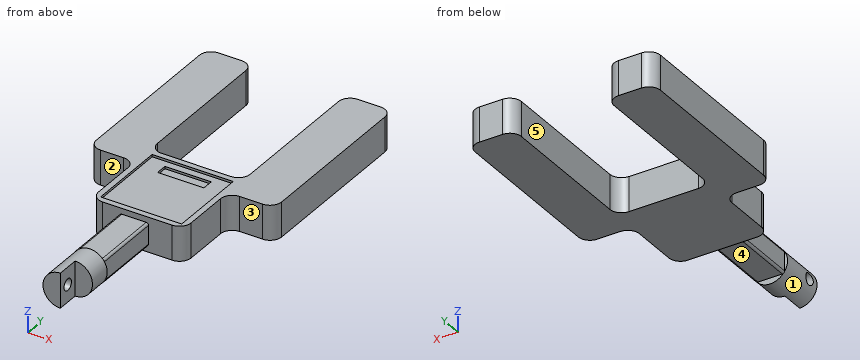
from build123d import *

# Parameters (mm, degrees)
SKETCH1_W           = 101.6
SKETCH1_H           = 101.6
BOSS_EXTRUDE1_DEPTH = 38.1
SKETCH2_W           = 50.8
SKETCH2_H           = 12.7
CUT_EXTRUDE1_DEPTH  = 5.08
SKETCH3_W           = 88.9
SKETCH3_H           = 88.9
CUT_EXTRUDE2_DEPTH  = 2.54
SKETCH4_W           = 31.75
SKETCH4_H           = 25.4
BOSS_EXTRUDE2_DEPTH = 76.2
SKETCH6_R           = 19.05
BOSS_EXTRUDE3_DEPTH = 50.8
SKETCH7_W           = 24.863041021
SKETCH7_H           = 49.917211664
CUT_EXTRUDE3_DEPTH  = 25.4
SKETCH8_W           = 50.8
SKETCH8_H           = 203.2
BOSS_EXTRUDE4_DEPTH = 38.1
FILLET1_R           = 12.7
SKETCH9_R           = 6.35
CUT_EXTRUDE4_DEPTH  = 301.990708903
FILLET2_R           = 2.54


with BuildPart() as part:
    # Sketch1 → Boss-Extrude1 (new body)
    with BuildSketch(Plane.XY):
        with Locations((50.8, 50.8)):
            Rectangle(SKETCH1_W, SKETCH1_H)
    extrude(amount=BOSS_EXTRUDE1_DEPTH)

    # Sketch2 → Cut-Extrude1 (cut)
    with BuildSketch(Plane.XY.offset(38.1)):
        with Locations((50.8, 80.942159742)):
            Rectangle(SKETCH2_W, SKETCH2_H)
    extrude(amount=-CUT_EXTRUDE1_DEPTH, mode=Mode.SUBTRACT)

    # Sketch3 → Cut-Extrude2 (cut)
    with BuildSketch(Plane.XY.offset(38.1)):
        with Locations((50.8, 50.8)):
            Rectangle(SKETCH3_W, SKETCH3_H)
    extrude(amount=-CUT_EXTRUDE2_DEPTH, mode=Mode.SUBTRACT)

    # Sketch4 → Boss-Extrude2 (add)
    with BuildSketch(Plane.XZ):
        with Locations((47.141096121, 19.05)):
            Rectangle(SKETCH4_W, SKETCH4_H)
    extrude(amount=BOSS_EXTRUDE2_DEPTH)

    # Sketch6 → Boss-Extrude3 (add)
    with BuildSketch(Plane.XZ.offset(76.2)):
        with Locations(Location((47.141096121, 19.05, 0), (0, 0, 138.189685104))):
            Circle(SKETCH6_R)
    extrude(amount=BOSS_EXTRUDE3_DEPTH)

    # Sketch7 → Cut-Extrude3 (cut)
    with BuildSketch(Plane.XZ.offset(127)):
        with Locations((59.572616632, 20.72754322)):
            Rectangle(SKETCH7_W, SKETCH7_H)
    extrude(amount=-CUT_EXTRUDE3_DEPTH, mode=Mode.SUBTRACT)

    # Sketch8 → Boss-Extrude4 (add)
    with BuildSketch(Plane(origin=(0, 0, 0), x_dir=(-1, 0, 0), z_dir=(0, 0, -1))):
        with Locations((25.4, 177.8)):
            Rectangle(SKETCH8_W, SKETCH8_H)
        with Locations((-127, 177.8)):
            Rectangle(SKETCH8_W, SKETCH8_H)
    extrude(amount=-BOSS_EXTRUDE4_DEPTH)

    # Fillet1
    fillet1_edges = [part.edges().sort_by_distance(p)[0] for p in [
        (101.6, 0, 19.05),
        (0, 0, 19.05),
        (0, 76.2, 19.05),
        (101.6, 76.2, 19.05),
        (101.6, 101.6, 19.05),
        (0, 101.6, 19.05),
        (152.4, 76.2, 19.05),
        (-50.8, 76.2, 19.05),
        (-50.8, 279.4, 19.05),
        (101.6, 279.4, 19.05),
        (152.4, 279.4, 19.05),
        (0, 279.4, 19.05),
    ]]
    fillet(fillet1_edges, radius=FILLET1_R)

    # Sketch9 → Cut-Extrude4 (cut, through all)
    with BuildSketch(Plane(origin=(47.141096121, 0, 0), x_dir=(0, 0, -1), z_dir=(1, 0, 0))):
        with Locations((-19.05, -114.3)):
            Circle(SKETCH9_R)
    extrude(amount=-CUT_EXTRUDE4_DEPTH, mode=Mode.SUBTRACT)

    # Fillet2
    # the kernel refuses this fillet: 2.54 mm, written as the material it takes off along each edge
    with BuildSketch(Plane(origin=(31.266096121, 0, 31.75), x_dir=(1, 0, 0), z_dir=(0, -1, 0))) as fillet2_piece_1:
        with BuildLine():
            CenterArc((FILLET2_R, -FILLET2_R), FILLET2_R, 90, 90)
            Line((0, -FILLET2_R), (0, 0))
            Line((0, 0), (FILLET2_R, 0))
        make_face()
    extrude(amount=76.2, mode=Mode.SUBTRACT)
    with BuildSketch(Plane(origin=(31.266096121, 0, 6.35), x_dir=(1, 0, 0), z_dir=(0, -1, 0)), Plane(origin=(63.016096121, 0, 6.35), x_dir=(0, 0, 1), z_dir=(0, -1, 0)), Plane(origin=(63.016096121, 0, 31.75), x_dir=(-1, 0, 0), z_dir=(0, -1, 0))) as fillet2_piece_2:
        with BuildLine():
            CenterArc((FILLET2_R, FILLET2_R), FILLET2_R, 180, 90)
            Line((0, FILLET2_R), (0, 0))
            Line((0, 0), (FILLET2_R, 0))
        make_face()
    extrude(amount=76.2, mode=Mode.SUBTRACT)


solid = part.part
The listing builds one solid part. Answer for the finished solid, in the listing's coordinates (mm). Face numbers are marked on the shaded views. A direction names the side the tool comes from. Coordinates: 2 decimals unless noted, no trailing zeros. Write each loop counter-clockwise with the first axis right and the second up, starting at its lowest first coordinate (ties: lowest second). Pieces come first, ordered by that corner, then holes. Notation, with made-up numbers: (-16, -7) - (-11, -7) arc R24 cw to (-11, 8) - close; hole circle Ø9 at (-11, 47). An arc over 180 degrees is marked (long way). Put each result on its own line as item: value.
1. The part is cut by section C-C on y = -18. Give the vertices of the cut face in (x, z), plus the area to 3 significant figures.
Answer sheet:
outline: (31.27, 8.89) arc R2.54 ccw to (33.81, 6.35) - (60.48, 6.35) arc R2.54 ccw to (63.02, 8.89) - (63.02, 29.21) arc R2.54 ccw to (60.48, 31.75) - (33.81, 31.75) arc R2.54 ccw to (31.27, 29.21) - close
area: 801 mm^2
2. A tool of negligible diameter and unlimited length cuts with its end or side. For the marked faces 1, 2, 3, 4 and 5, from which of +Z, -Z, +X, -X, +Y, -Y can it reach the whole face along a straight path? Write none if from no direction.
Answer sheet:
face 1: -Y
face 2: +Z, -Z, -X, -Y
face 3: +Z, -Z, +X, -Y
face 4: -Z, +X, -X
face 5: +Z, -Z, +Y
3. The part is cut by section A-A on y = 211. Give the vertices of the cut face in (x, z).
Answer sheet:
outline: (-50.8, 0) - (0, 0) - (0, 38.1) - (-50.8, 38.1) - close; (101.6, 0) - (152.4, 0) - (152.4, 38.1) - (101.6, 38.1) - close
4. The part is cut by section D-D on y = -114.3. Give the vertices of the cut face in (x, z).
Answer sheet:
outline: (29.18, 12.7) arc R19.05 ccw to (47.14, 0) - (47.14, 12.7) - close; (29.18, 25.4) - (47.14, 25.4) - (47.14, 38.1) arc R19.05 ccw to start
5. Flat-ended cylindrical pins translate along their axes: pin 1 Ø3 at (x, z) = (12, 28) entering from +Y; pin 2 Ø1.3 at (x, z) = (58, 34.5) entering from -Y; pin 3 Ø8 at (x, z) = (91, 32) entering from +Y; pin 4 Ø3 at (x, y) = (-30, 193.5) entering from -Z. Find the tip coordinate at first contact, or state that the pin passes through.
Answer sheet:
pin 1: stops at y = 101.79
pin 2: stops at y = -101.6
pin 3: stops at y = 103.16
pin 4: stops at z = 0
6. Find the intervals of material crossed by line 1 along X through (y, z) = (210.5, 27); line 2 along Y through (x, z) = (38, 19.05); line 3 along X through (y, z) = (28, 14), in increasing order. Write a range as from..to.
Answer sheet:
line 1: x = -50.8..0, 101.6..152.4
line 2: y = -127..-120.65, -107.95..101.6
line 3: x = 0..101.6
7. The part is cut by section B-B on x = 52. Give the vertices of the cut face in (y, z), plus the area to 3 significant figures.
Answer sheet:
outline: (-101.6, 0.63) - (-76.2, 0.63) - (-76.2, 6.35) - (0, 6.35) - (0, 0) - (101.6, 0) - (101.6, 38.1) - (95.25, 38.1) - (95.25, 35.56) - (87.29, 35.56) - (87.29, 33.02) - (74.59, 33.02) - (74.59, 35.56) - (6.35, 35.56) - (6.35, 38.1) - (0, 38.1) - (0, 31.75) - (-76.2, 31.75) - (-76.2, 37.47) - (-101.6, 37.47) - close
area: 6,480 mm^2
